Here's how the part is built. I have some questions about the finished solid (model axes, mm). Give positions to 0.01 mm unless a question says otherwise; leave off trailing zeros. Loops run counter-clockwise (first coordinate to the right, second up) from the corner with the lowest first, then second, coordinate; pieces in that order, holes last. Notation, with made-up numbers: (-23.75, -20.75) - (-6.75, -20.75) arc R25 cw to (-6.75, 12.25) - close; hole circle Ø8 at (68, 57). An arc over 180 degrees is marked (long way). Use one line per item in the form item = value.
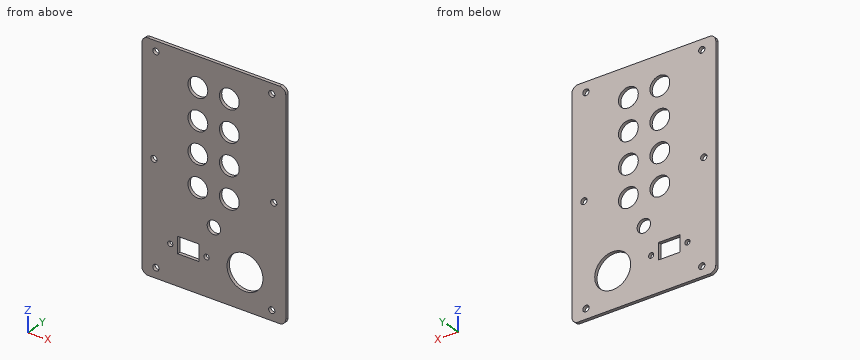
from build123d import *

# Parameters (mm, degrees)
SKETCH1_W           = 114.3
SKETCH1_H           = 177.8
SKETCH1_R           = 7.874
SKETCH1_R_2         = 5.334
SKETCH1_R_3         = 14.2875
SKETCH1_R_4         = 2.4892
SKETCH1_R_5         = 2.06375
SKETCH1_W_2         = 17.018
SKETCH1_H_2         = 13.081
BOSS_EXTRUDE1_DEPTH = 2.54
FILLET1_R           = 4.92


with BuildPart() as part:
    # Sketch1 → Boss-Extrude1 (new body)
    with BuildSketch(Plane(origin=(0, 0, 0), x_dir=(1, 0, 0), z_dir=(0, 1, 0))):
        with Locations((0, 12.933192571)):
            Rectangle(SKETCH1_W, SKETCH1_H)
        with Locations(Location((-12.7, 22.458192571, 0), (0, 0, 270))):
            Circle(SKETCH1_R, mode=Mode.SUBTRACT)
        with Locations(Location((0, 47.858192571, 0), (0, 0, 270))):
            Circle(SKETCH1_R_2, mode=Mode.SUBTRACT)
        with Locations(Location((24.765, 72.940692571, 0), (0, 0, 270))):
            Circle(SKETCH1_R_3, mode=Mode.SUBTRACT)
        with Locations(Location((-46.0375, -68.029307429, 0), (0, 0, 270))):
            Circle(SKETCH1_R_4, mode=Mode.SUBTRACT)
        with Locations(Location((-46.0375, 93.895692571, 0), (0, 0, 270))):
            Circle(SKETCH1_R_4, mode=Mode.SUBTRACT)
        with Locations(Location((-47.625, 12.933192571, 0), (0, 0, 270))):
            Circle(SKETCH1_R_4, mode=Mode.SUBTRACT)
        with Locations(Location((46.0375, 93.895692571, 0), (0, 0, 90))):
            Circle(SKETCH1_R_4, mode=Mode.SUBTRACT)
        with Locations(Location((47.625, 12.933192571, 0), (0, 0, 90))):
            Circle(SKETCH1_R_4, mode=Mode.SUBTRACT)
        with Locations(Location((46.0375, -68.029307429, 0), (0, 0, 90))):
            Circle(SKETCH1_R_4, mode=Mode.SUBTRACT)
        with Locations(Location((-5.801987124, 72.035346476, 0), (0, 0, 270))):
            Circle(SKETCH1_R_5, mode=Mode.SUBTRACT)
        with Locations(Location((-34.630987124, 72.035346476, 0), (0, 0, 90))):
            Circle(SKETCH1_R_5, mode=Mode.SUBTRACT)
        with Locations(Location((12.3, 22.458192571, 0), (0, 0, 270))):
            Circle(SKETCH1_R, mode=Mode.SUBTRACT)
        with Locations(Location((12.3, -2.541807429, 0), (0, 0, 270))):
            Circle(SKETCH1_R, mode=Mode.SUBTRACT)
        with Locations(Location((12.3, -27.541807429, 0), (0, 0, 270))):
            Circle(SKETCH1_R, mode=Mode.SUBTRACT)
        with Locations(Location((12.3, -52.541807429, 0), (0, 0, 270))):
            Circle(SKETCH1_R, mode=Mode.SUBTRACT)
        with Locations(Location((-12.7, -2.541807429, 0), (0, 0, 270))):
            Circle(SKETCH1_R, mode=Mode.SUBTRACT)
        with Locations(Location((-12.7, -27.541807429, 0), (0, 0, 270))):
            Circle(SKETCH1_R, mode=Mode.SUBTRACT)
        with Locations(Location((-12.7, -52.541807429, 0), (0, 0, 270))):
            Circle(SKETCH1_R, mode=Mode.SUBTRACT)
        with Locations((-20.216487124, 70.907248902)):
            Rectangle(SKETCH1_W_2, SKETCH1_H_2, mode=Mode.SUBTRACT)
    extrude(amount=BOSS_EXTRUDE1_DEPTH)

    # Fillet1
    fillet1_edges = [part.edges().sort_by_distance(p)[0] for p in [
        (-57.15, 1.27, -101.833192571),
        (57.15, 1.27, -101.833192571),
        (57.15, 1.27, 75.966807429),
        (-57.15, 1.27, 75.966807429),
    ]]
    fillet(fillet1_edges, radius=FILLET1_R)


solid = part.part
(1) If we section it at D-D (y = 1.05): Give the number of separate pieces and of enclosed holes in the cut face, plus the area to 3 significant figures.
Geometry says:
separate_pieces = 1
enclosed_holes = 19
area = 17,600 mm²
(2) If we section it at A-A (z = 1): List the corners of the cut face in (x, y) for me, plus the area to 3 significant figures.
Geometry says:
outline = (-57.15, 0) - (-20.42, 0) - (-20.42, 2.54) - (-57.15, 2.54) - close; (-4.98, 0) - (4.58, 0) - (4.58, 2.54) - (-4.98, 2.54) - close; (20.02, 0) - (57.15, 0) - (57.15, 2.54) - (20.02, 2.54) - close
area = 212 mm²
(3) If we section it at B-B (x = 37): List the corners of the cut face in (y, z) for me.
Geometry says:
outline = (0, -101.83) - (2.54, -101.83) - (2.54, -80.32) - (0, -80.32) - close; (0, -65.56) - (2.54, -65.56) - (2.54, 75.97) - (0, 75.97) - close
(4) For P1, Ø9.5, axis at x = 12.3, z = 2.54, coming from the -Y side, with a flat end and sliding along its axis, tell me the tip position at first contact or that it passes through.
Geometry says:
P1 = through
(5) If I drill on probe 1 along X at (y, z) = (1.15, 55.5); probe 2 along X at (y, z) = (0.4, -93.5); probe 3 along Z at (x, y) = (15, 1.3), over which ranges is the centre line in solid material (lowest first)?
Geometry says:
probe_1 = -57.15 to -20, -5.4 to 5, 19.6 to 57.15
probe_2 = -57.15 to -48.5, -43.58 to 43.58, 48.5 to 57.15
probe_3 = -101.83 to -83.37, -62.51 to -29.85, -15.06 to -4.85, 9.94 to 20.15, 34.94 to 45.15, 59.94 to 75.97
(6) If we section it at C-C (z = -83.5): List the corners of the cut face in (x, y) for me, plus the area to 3 significant figures.
Geometry says:
outline = (-57.15, 0) - (15.14, 0) - (15.14, 2.54) - (-57.15, 2.54) - close; (34.39, 0) - (57.15, 0) - (57.15, 2.54) - (34.39, 2.54) - close
area = 241 mm²
